Input: dimensioned drawing with shaded views. Units: mm. Origin: part minimum x, y, z. Round coordinates to 2 decimals unless told otherwise and drop trailing zeros. Loops run counter-clockwise (first coordinate to the right, second up) from the corner with the lowest first, then second, coordinate; pieces in that order, holes last. Notation, with made-up numbers: (38.25, -25) - (79.25, -25) arc R16 ccw to (79.25, -11) - close; hole circle Ø9 at (-11, 86). An arc over 180 degrees is marked (long way). Answer as a JSON object with one key per item and string values. Group by question number.
Item 1: Line query: line 1 (Y direction, x = 12, z = 2); line 2 (Y direction, x = 14, z = 7); line 3 (Y direction, x = 5, z = 7.5). Output: solid intervals per line, ascending.
Item 2: Section A-A (z = 7). Return the cut outline in (x, y).
Item 3: Section B-B (x = 12). Return the cut outline in (y, z).
Item 4: Section D-D (x = 2). Return the cut outline in (y, z), plus the area to 3 significant figures.
Item 5: Section C-C (y = 50). Return the cut outline in (x, z), plus the area to 3 significant figures.
Item 6: First-contact query: pin 1 (5 mm diameter, centred on x = 12, y = 48, fed in from +Z); pin 2 (4 mm diameter, centred on x = 20.5, z = 4.5, fed in from -Y). Flat tips, straight axial feed; report the tip coordinate or a pass-through.
Item 7: Draft query along Y for the marked faces 1, 2 and 3. Return one class per face: released by +Y, released by -Y, zero draft, split by the parting line, or undercut.
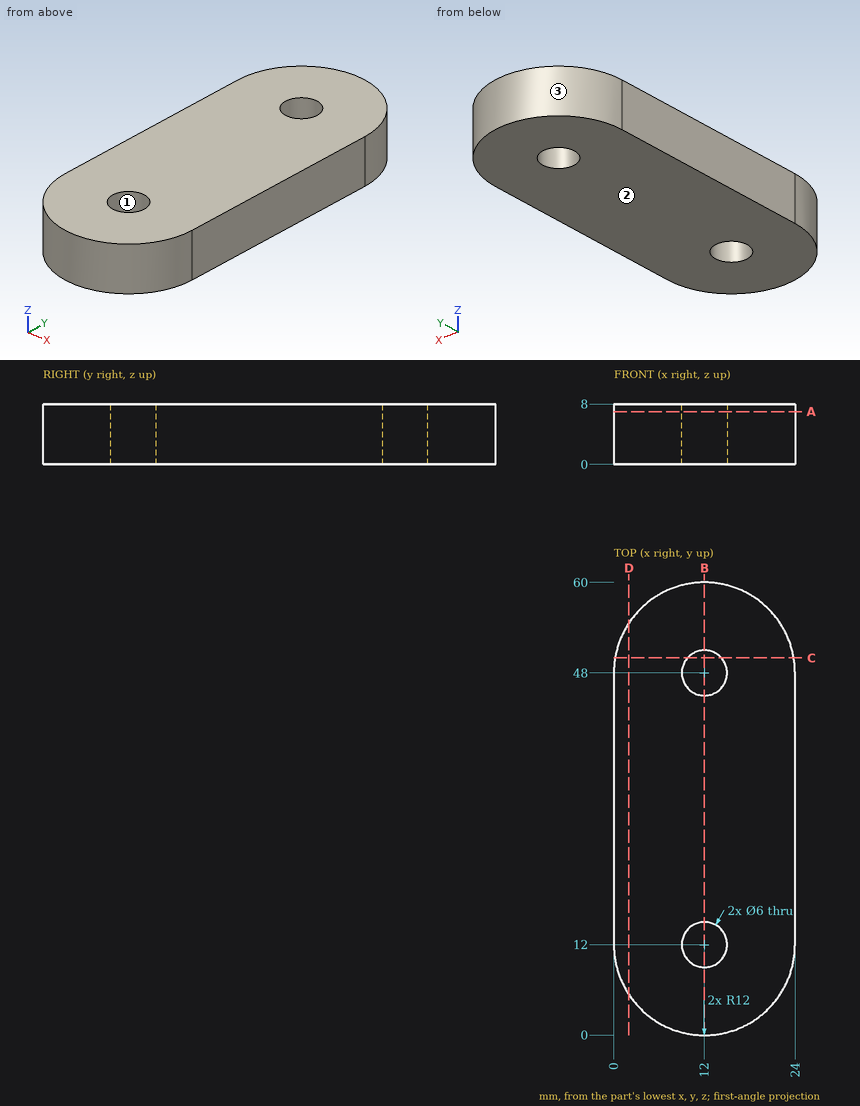
Values:
{
 "1": {"line 1": "y = 0 to 9, 15 to 45, 51 to 60", "line 2": "y = 0.17 to 9.76, 14.24 to 45.76, 50.24 to 59.83", "line 3": "y = 2.25 to 57.75"},
 "2": {"outline": "(0, 12) arc R12 ccw to (24, 12) - (24, 48) arc R12 ccw to (0, 48) - close; hole circle Ø6 at (12, 12); hole circle Ø6 at (12, 48)"},
 "3": {"outline": "(0, 0) - (9, 0) - (9, 8) - (0, 8) - close; (15, 0) - (45, 0) - (45, 8) - (15, 8) - close; (51, 0) - (60, 0) - (60, 8) - (51, 8) - close"},
 "4": {"outline": "(5.37, 0) - (54.63, 0) - (54.63, 8) - (5.37, 8) - close", "area": "394 mm^2"},
 "5": {"outline": "(0.17, 0) - (9.76, 0) - (9.76, 8) - (0.17, 8) - close; (14.24, 0) - (23.83, 0) - (23.83, 8) - (14.24, 8) - close", "area": "154 mm^2"},
 "6": {"pin 1": "passes through", "pin 2": "stops at y = 1.91"},
 "7": {"face 1": "undercut", "face 2": "zero draft", "face 3": "released by +Y"}
}
